Verification items for this drawing (mm, ordinates from the low corner). Give positions to 0.01 mm unless a question says otherwise; leave off trailing zeros. Write each loop counter-clockwise with the first axis right and the second up, starting at its lowest first coordinate (ties: lowest second). Pieces come first, ordered by that corner, then holes. Notation, with made-up numbers: (-28.75, -32) -> (17.25, -32) arc R19 ccw to (17.25, -17) -> close; hole circle Ø1 at (57.5, 80.25). An arc over 180 degrees is marked (long way). Use one line per item in the form item = value. Start each with the question number.
(1) Section check B-B, the plane y = 34.5. Record the cut outline in (x, z).
(2) Section check C-C, the plane x = 25. Record the cut outline in (y, z), plus the area to 3 significant figures.
(3) Depth check by flat-ended pin: pin 1 Ø5.5 at (x, y) = (5, 7.5) entering from -Z. Enter the tip coordinate at first touch or a pass-through.
(4) Scan lines: L1, parallel to Y at x = 25, z = 0.65; L2, parallel to Y at x = 6.5, z = 2.6; L3, parallel to Y at x = 20, z = 1.75. Record each from-to range of solid material in increasing order.
(5) Section check A-A, the plane y = 61.5. Record the cut outline in (x, z).
(6) Section check D-D, the plane z = 1.65. Record the cut outline in (x, y), plus the area to 3 significant figures.
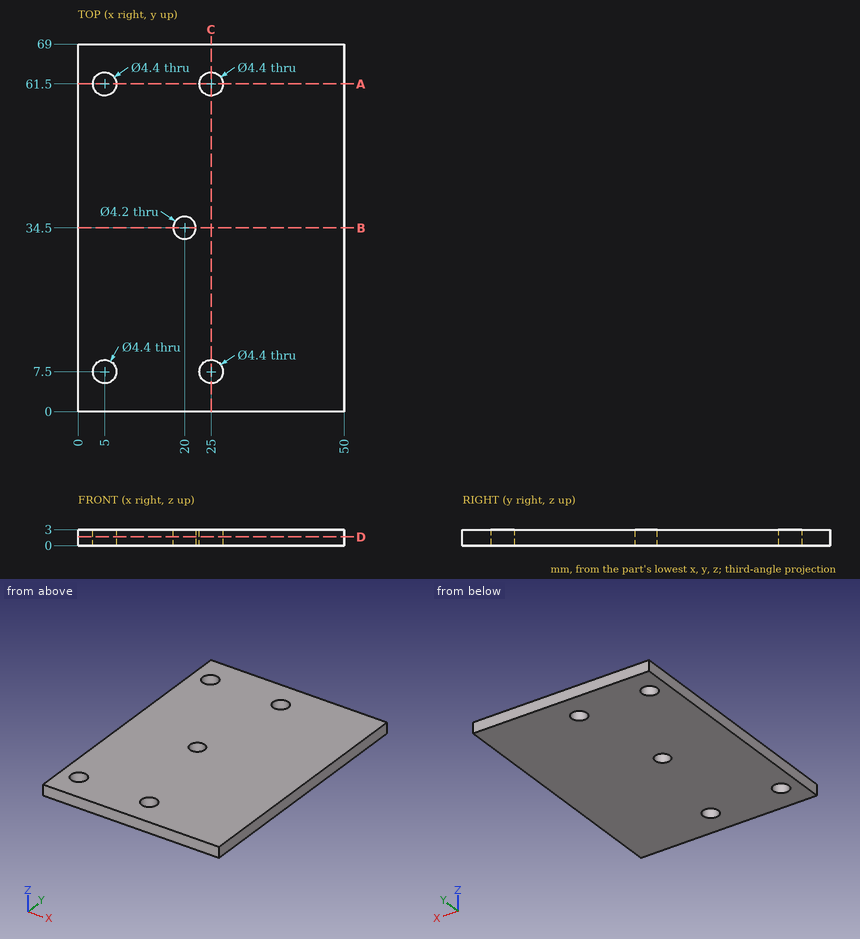
Completed:
q1.outline = (0, 0) -> (17.9, 0) -> (17.9, 3) -> (0, 3) -> close; (22.1, 0) -> (50, 0) -> (50, 3) -> (22.1, 3) -> close
q2.outline = (0, 0) -> (5.3, 0) -> (5.3, 3) -> (0, 3) -> close; (9.7, 0) -> (59.3, 0) -> (59.3, 3) -> (9.7, 3) -> close; (63.7, 0) -> (69, 0) -> (69, 3) -> (63.7, 3) -> close
q2.area = 181 mm²
q3.pin_1 = 0
q4.L1 = 0 to 5.3, 9.7 to 59.3, 63.7 to 69
q4.L2 = 0 to 5.89, 9.11 to 59.89, 63.11 to 69
q4.L3 = 0 to 32.4, 36.6 to 69
q5.outline = (0, 0) -> (2.8, 0) -> (2.8, 3) -> (0, 3) -> close; (7.2, 0) -> (22.8, 0) -> (22.8, 3) -> (7.2, 3) -> close; (27.2, 0) -> (50, 0) -> (50, 3) -> (27.2, 3) -> close
q6.outline = (0, 0) -> (50, 0) -> (50, 69) -> (0, 69) -> close; hole circle Ø4.4 at (5, 7.5); hole circle Ø4.4 at (5, 61.5); hole circle Ø4.2 at (20, 34.5); hole circle Ø4.4 at (25, 7.5); hole circle Ø4.4 at (25, 61.5)
q6.area = 3,380 mm²
